Here's the drawing with two shaded views (mm, measured from the low corner). I have some questions. A direction names the side the tool comes from. Give positions to 0.01 mm unless a question says otherwise; leave off trailing zeros. Loops run counter-clockwise (first coordinate to the right, second up) from the corner with the lowest first, then second, coordinate; pieces in that order, holes last. Notation, with made-up numbers: M 88,4 L 111,4 A12 cw 111,27 Z; hole C 63.5,8 d11. An arc over 180 degrees is marked long. Use a Markdown table: item, result. Add a question column.
1) Suppose I cut it at C-C on x = 236.5. List the corners of the cut face in (y, z) for me, and give its area (3 significant figures).
2) If I drill on line 1 along X through (y, z) = (3.5, 15); line 2 along Z through (x, y) = (15, 5); line 3 along X through (y, z) = (19.75, 22.75), over which ranges is the centre line in solid material (lowest first)? Write a range as [from, to].
3) Will these pins go through, and if not, where does the flat tip stop? pin 1 Ø3 at (x, y) = (159.5, 11) entering from -Z; pin 2 Ø2.5 at (x, z) = (255, 15) entering from +Y.
4) Which directions (+Z, -Z, +X, -X, +Y, -Y) give clear straight access to the entire face, cutting with the end or side of a thin tool? Please do the marked faces 1, 2 and 3.
5) Suppose I cut it at B-B on y = 16. List the corners of the cut face in (x, z) for me.
6) Suppose I cut it at A-A on z = 7.25. List the corners of the cut face in (x, y) for me, and give its area (4 significant figures).
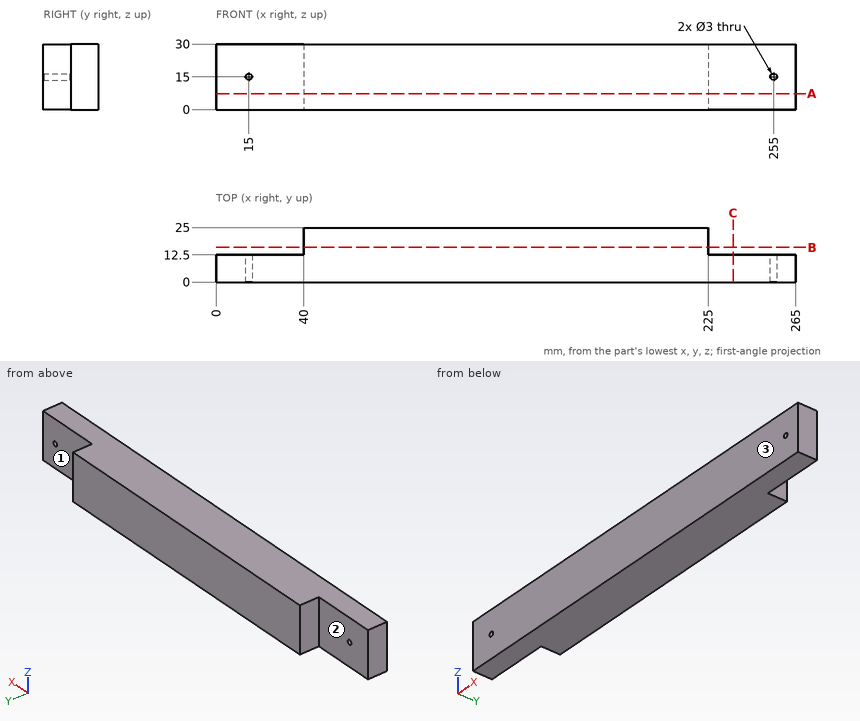
Answer block:
| question | item | result |
|---|---|---|
| 1 | outline | M 0,0 L 12.5,0 L 12.5,30 L 0,30 Z |
| 1 | area | 375 mm^2 |
| 2 | line 1 | x = [0, 13.5], [16.5, 253.5], [256.5, 265] |
| 2 | line 2 | z = [0, 13.5], [16.5, 30] |
| 2 | line 3 | x = [40, 225] |
| 3 | pin 1 | stops at z = 0 |
| 3 | pin 2 | passes through |
| 4 | face 1 | +Z, -Z, +X, +Y |
| 4 | face 2 | +Z, -Z, -X, +Y |
| 4 | face 3 | +Z, -Z, +X, -X, -Y |
| 5 | outline | M 40,0 L 225,0 L 225,30 L 40,30 Z |
| 6 | outline | M 0,0 L 265,0 L 265,12.5 L 225,12.5 L 225,25 L 40,25 L 40,12.5 L 0,12.5 Z |
| 6 | area | 5,625 mm^2 |
